Design review of the part built by this model. Coordinates are the model's own, in mm. Face numbers are marked on the shaded views. A direction names the side the tool comes from. Coordinates: 2 decimals unless noted, no trailing zeros. Write each loop counter-clockwise with the first axis right and the second up, starting at its lowest first coordinate (ties: lowest second). Pieces come first, ordered by that corner, then holes.
Q1. For pin 1 Ø9.5 at (y, z) = (-5, -49) entering from -X; pin 2 Ø5.5 at (y, z) = (-12, -66) entering from +X, all flat-tipped, find the tip position at first contact; note any pin that passes through.
Q2. For L1, parallel to X at y = -2, z = -82.5; L2, parallel to Z at x = 19, y = -8; L3, parallel to Z at x = -4.5, y = -7.5, list the stretches that pass through material, from the lowest coordinate up.
Q3. Take a section at A-A, the plane y = -12.75. Write out the cut boundary in (x, z) (3 decimals), plus the area to 3 significant figures.
Q4. Take a section at C-C, the plane x = 9. Write out the cut boundary in (y, z).
Q5. Take a section at B-B, the plane z = -97.5. Write out the cut boundary in (x, y), plus the area to 3 significant figures.
Q6. For the marked faces 1, 2 and 3, list the 3-axis set-ups (+Z, -Z, +X, -X, +Y, -Y) from which the entire face can be reached by the end or side of a thin tool; tool diameter is ignored.
from build123d import *

# Parameters (mm, degrees)
F1_DEPTH = 19.05


with BuildPart() as f1:
    # F0 (on Front) → F1 (new body)
    with BuildSketch(Plane.XZ):
        with BuildLine():
            Line((-17.78, -114.3), (17.78, -114.3))
            Line((17.78, -114.3), (17.78, -27.305))
            ThreePointArc((17.78, -27.305), (18.337962, -25.957962), (19.685, -25.4))
            Line((19.685, -25.4), (20.32, -25.4))
            ThreePointArc((20.32, -25.4), (21.667038, -24.842038), (22.225, -23.495))
            Line((22.225, -23.495), (22.225, 99.185287))
            ThreePointArc((22.225, 99.185287), (10.399365, 105.694035), (0, 114.3))
            ThreePointArc((0, 114.3), (-10.399365, 105.694035), (-22.225, 99.185287))
            Line((-22.225, 99.185287), (-22.225, -22.86))
            ThreePointArc((-22.225, -22.86), (-21.667038, -24.207038), (-20.32, -24.765))
            Line((-20.32, -24.765), (-19.685, -24.765))
            ThreePointArc((-19.685, -24.765), (-18.337962, -25.322962), (-17.78, -26.67))
            Line((-17.78, -26.67), (-17.78, -114.3))
        make_face()
    extrude(amount=F1_DEPTH)


solid = f1.part
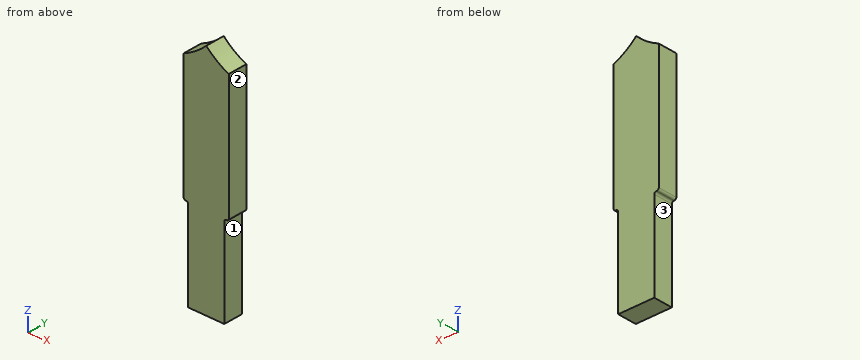
Responses:
1. pin 1: stops at x = -17.78
1. pin 2: stops at x = 17.78
2. L1: x = -17.78 to 17.78
2. L2: z = -25.53 to 100.68
2. L3: z = -114.3 to 110.17
3. outline: (-22.225, -22.86) arc R1.905 ccw to (-20.32, -24.765) - (-19.685, -24.765) arc R1.905 cw to (-17.78, -26.67) - (-17.78, -114.3) - (17.78, -114.3) - (17.78, -27.305) arc R1.905 cw to (19.685, -25.4) - (20.32, -25.4) arc R1.905 ccw to (22.225, -23.495) - (22.225, 99.185) arc R71.842 cw to (0, 114.3) arc R71.842 cw to (-22.225, 99.185) - close
3. area: 8,990 mm2
4. outline: (-19.05, -114.3) - (0, -114.3) - (0, 106.67) - (-19.05, 106.67) - close
5. outline: (-17.78, -19.05) - (17.78, -19.05) - (17.78, 0) - (-17.78, 0) - close
5. area: 677 mm2
6. face 1: -Z, +X, +Y, -Y
6. face 2: +Z, -Z, +X, +Y, -Y
6. face 3: -Z, -X, +Y, -Y
